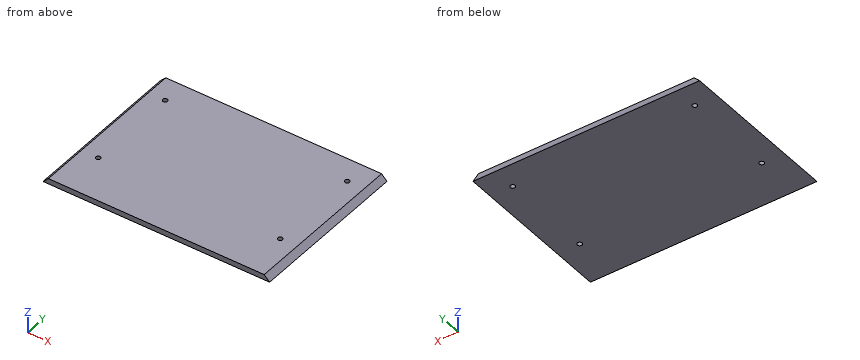
Autodesk Inventor part; units mm, degrees
ref_plane "YZ Plane" through (0, 0, 0) normal (1, 0, 0) x (0, 1, 0)
ref_plane "XZ Plane" through (0, 0, 0) normal (0, 1, 0) x (-1, 0, 0)
ref_plane "XY Plane" through (0, 0, 0) normal (0, 0, 1) x (1, 0, 0)
sketch "Sketch1" plane through (0, 0, 0) normal (0, 0, 1) x (1, 0, 0)
  line L0 (0, 0) -> (168, 0)
  line L1 (168, 0) -> (168, -121)
  line L2 (168, -121) -> (0, -121)
  line L3 (0, -121) -> (0, 0)
  dimension "d0" = 168
  dimension "d1" = 121
extrude "Extrusion1" add sketch "Sketch1" along normal blind 4
sketch "Sketch2" plane through (0, 0, 0) normal (0, 0, -1) x (-1, 0, 0)
  line L0 (0, -121) -> (-168, -121)
  line L1 (0, -121) -> (-16.5, -121)
  line L2 (-16.5, -121) -> (-16.5, -87)
  line L3 (-16.5, -87) -> (0, -87)
  line L4 (0, -87) -> (0, -121)
  point P0 (0, 0)
  dimension "d4" = 16.5
  dimension "d5" = 34
hole "Hole1" at (16.5, -87, 0) direction (0, 0, 1) diameter 3.5 depth 8.8
ref_plane "Work Plane1" through (84, -121, 0) normal (-1, 0, 0) x (0, 0, 1)
ref_plane "Work Plane2" through (0, -60.5, 0) normal (0, 1, 0) x (1, 0, 0)
sketch "Sketch3" plane through (0, 0, 4) normal (0, 0, 1) x (1, 0, 0)
  line L0 (168, 0) -> (0, 0)
  line L1 (0, 0) -> (16.5, 0)
  line L2 (16.5, 0) -> (16.5, -18)
  line L3 (16.5, -18) -> (0, -18)
  line L4 (0, -18) -> (0, 0)
  dimension "d13" = 16.5
  dimension "d14" = 18
hole "Hole2" at (16.5, -18, 4) direction (0, 0, -1) diameter 3.5 depth 8.8
mirror "Mirror1" about plane through (84, -121, 0) normal (-1, 0, 0) of "Hole2", "Hole1"
chamfer "Chamfer1" distance 4 angle 45 2 edges at (0, -60.5, 4) (168, -60.5, 4)
properties part number "wall-left"
The listing builds one solid part. Answer for the finished solid, in the listing's coordinates (mm). Give positions to 0.01 mm unless a question says otherwise; leave off trailing zeros. Write each loop counter-clockwise with the first axis right and the second up, starting at its lowest first coordinate (ties: lowest second). Pieces come first, ordered by that corner, then holes. Notation, with made-up numbers: (24, 12) - (57, 12) arc R12 ccw to (57, 32) - close; hole circle Ø3 at (-21.75, 29.25). An arc over 180 degrees is marked (long way). One line per question, with ' | ' between items. Start each with the question number.
1. Section A-A, the plane y = -87 is taken. Count the separate pieces of the cut face and the enclosed holes in it, then the cut area to 3 significant figures.
2. Section C-C, the plane z = 3.15 is taken. Determine the outline of the cut face in (x, y).
3. Section B-B, the plane x = 151.5 is taken. Determine the outline of the cut face in (y, z), then the cut area to 3 significant figures.
4. Straight lines are drawn through the part: line 1 (Y direction, x = 151.5, z = 1.2); line 2 (X direction, y = -18, z = 1.1); line 3 (X direction, y = -18, z = 1.7). For each, find the intervals that lie inside material, in ascending order.
5. Given P1, Ø1, axis at y = -77, z = 1, coming from the -X side; P2, Ø1, axis at y = -23, z = 1.5, coming from the -X side, each flat-ended and moving along its own axis, determine where each tip first touches the part or whether it passes through.
Result:
1) separate pieces: 3 | enclosed holes: 0 | area: 628 mm2
2) outline: (3.15, -121) - (164.85, -121) - (164.85, 0) - (3.15, 0) - close; hole circle Ø3.5 at (16.5, -87); hole circle Ø3.5 at (16.5, -18); hole circle Ø3.5 at (151.5, -87); hole circle Ø3.5 at (151.5, -18)
3) outline: (-121, 0) - (-88.75, 0) - (-88.75, 4) - (-121, 4) - close; (-85.25, 0) - (-19.75, 0) - (-19.75, 4) - (-85.25, 4) - close; (-16.25, 0) - (0, 0) - (0, 4) - (-16.25, 4) - close | area: 456 mm2
4) line 1: y = -121 to -88.75, -85.25 to -19.75, -16.25 to 0 | line 2: x = 1.1 to 14.75, 18.25 to 149.75, 153.25 to 166.9 | line 3: x = 1.7 to 14.75, 18.25 to 149.75, 153.25 to 166.3
5) P1: stops at x = 0.5 | P2: stops at x = 1
